Model file for the job. Use its own axes, mm. Face numbers are marked on the shaded views. A direction names the side the tool comes from. Coordinates: 2 decimals unless noted, no trailing zeros. Loops run counter-clockwise (first coordinate to the right, second up) from the corner with the lowest first, then second, coordinate; pieces in that order, holes last.
Autodesk Inventor part; units mm, degrees
ref_plane "YZ Plane" through (0, 0, 0) normal (1, 0, 0) x (0, 1, 0)
ref_plane "XZ Plane" through (0, 0, 0) normal (0, 1, 0) x (-1, 0, 0)
ref_plane "XY Plane" through (0, 0, 0) normal (0, 0, 1) x (1, 0, 0)
sketch "Sketch1" plane through (0, 0, 0) normal (0, 0, 1) x (1, 0, 0)
  line L0 (0, 0) -> (525.78, 0)
  line L1 (0, 0) -> (0, 101.6)
  line L2 (0, 101.6) -> (262.89, 253.3796)
  line L3 (262.89, 253.3796) -> (525.78, 101.6)
  line L4 (525.78, 101.6) -> (525.78, 0)
  line L5 (262.89, 246.0473) -> (6.35, 97.9338)
  line L6 (6.35, 97.9338) -> (6.35, 6.35)
  line L7 (6.35, 6.35) -> (519.43, 6.35)
  line L8 (519.43, 6.35) -> (519.43, 97.9338)
  line L9 (519.43, 97.9338) -> (262.89, 246.0473)
  point P0 (262.89, 0)
  dimension "d0" = 525.78
  dimension "d1" = 101.6
  dimension "d2" = 120
  dimension "d3" = 6.35
extrude "Extrusion1" add sketch "Sketch1" along normal blind 355.6
sketch "Sketch2" plane through (0, 0, 355.6) normal (0, 0, 1) x (1, 0, 0)
  line L0 (262.89, 246.0473) -> (519.43, 97.9338)
  line L1 (519.43, 97.9338) -> (519.43, 6.35)
  line L2 (519.43, 6.35) -> (6.35, 6.35)
  line L3 (6.35, 6.35) -> (6.35, 97.9338)
  line L4 (6.35, 97.9338) -> (262.89, 246.0473)
  line L5 (0, 0) -> (525.78, 0)
  line L6 (525.78, 0) -> (525.78, 101.6)
  line L7 (525.78, 101.6) -> (262.89, 253.3796)
  line L8 (262.89, 253.3796) -> (0, 101.6)
  line L9 (0, 101.6) -> (0, 0)
  circle A0 centre (262.89, 121.3796) radius 60
  dimension "d6" = 120
  dimension "d7" = 132
extrude "Extrusion2" add sketch "Sketch2" along normal blind 6.35 contours L0 L1 L2 L3 L4 | L9 L8 L7 L6 L5
sketch "Sketch3" plane through (0, 0, 0) normal (0, -1, 0) x (1, 0, 0)
  line L0 (0, 0) -> (525.78, 0) construction
  line L1 (525.78, 0) -> (525.78, 88.9)
  line L2 (525.78, 88.9) -> (0, 88.9) construction
  line L3 (0, 88.9) -> (0, 0) construction
  line L4 (86.36, 21.95) -> (86.36, 66.95) construction
  circle A0 centre (86.36, 44.45) radius 2.3812
  circle A1 centre (86.36, 21.95) radius 2.3812
  circle A2 centre (86.36, 66.95) radius 2.3812
  line L5 (146.36, 49.45) -> (146.36, 29.45) construction
  line L6 (156.36, 66.95) -> (156.36, 21.95) construction
  line L7 (146.36, 29.45) -> (166.36, 29.45) construction
  line L8 (166.36, 49.45) -> (146.36, 49.45) construction
  line L9 (86.36, 66.95) -> (226.36, 66.95) construction
  line L10 (226.36, 21.95) -> (86.36, 21.95) construction
  line L11 (86.36, 44.45) -> (226.36, 44.45) construction
  line L12 (166.36, 29.45) -> (166.36, 49.45) construction
  line L13 (226.36, 66.95) -> (226.36, 21.95) construction
  circle A3 centre (226.36, 66.95) radius 2.3813
  circle A4 centre (226.36, 44.45) radius 2.3813
  circle A5 centre (226.36, 21.95) radius 2.3813
  circle A6 centre (156.36, 39.45) radius 10
  line L14 (0, 0) -> (0, 361.95)
  line L15 (525.78, 0) -> (525.78, 361.95)
  line L16 (0, 0) -> (525.78, 0)
  point P0 (0, 44.45)
  point P1 (146.36, 39.45)
  point P2 (166.36, 39.45)
  point P3 (262.89, 0)
  dimension "d10" = 45
  dimension "d11" = 140
  dimension "d12" = 4.7625
  dimension "d13" = 4.7625
  dimension "d14" = 4.7625
  dimension "d15" = 4.7625
  dimension "d16" = 4.7625
  dimension "d17" = 4.7625
  dimension "d18" = 60
  dimension "d19" = 7.5
  dimension "d20" = 20
  dimension "d21" = 20
  dimension "d22" = 86.36
  dimension "d23" = 88.9
extrude "Extrusion3" cut sketch "Sketch3" against normal blind 6.35
sketch "Sketch4" plane through (0, 0, 0) normal (0, -1, 0) x (1, 0, 0)
  line L0 (71.36, 0) -> (241.36, 0)
  line L1 (241.36, 0) -> (241.36, 85)
  line L2 (241.36, 85) -> (71.36, 85)
  line L3 (71.36, 85) -> (71.36, 0)
  line L4 (0, 0) -> (525.78, 0) construction
  circle A0 centre (156.36, 39.45) radius 10 construction
  point P0 (156.36, 85)
  dimension "d26" = 170
  dimension "d27" = 85
extrude "Extrusion4" cut sketch "Sketch4" against normal blind 6.35
sketch "Sketch5" plane through (0, 0, 361.95) normal (0, -1, 0) x (1, 0, 0)
  line L0 (519.43, -6.35) -> (6.35, -6.35)
  line L1 (241.36, -361.95) -> (525.78, -361.95)
  line L2 (0, -361.95) -> (0, 0)
  line L3 (525.78, -361.95) -> (0, -361.95)
  line L4 (0, -361.95) -> (0, -243.4167)
  line L5 (0, -243.4167) -> (525.78, -243.4167)
  line L6 (525.78, -243.4167) -> (525.78, -361.95)
  line L7 (525.78, -243.4167) -> (0, -243.4167)
  line L8 (0, -243.4167) -> (0, -124.8833)
  line L9 (0, -124.8833) -> (525.78, -124.8833)
  line L10 (525.78, -124.8833) -> (525.78, -243.4167)
  line L11 (525.78, -124.8833) -> (0, -124.8833)
  line L12 (0, -124.8833) -> (0, 0)
  line L13 (0, 0) -> (525.78, 0)
  line L14 (525.78, 0) -> (525.78, -124.8833)
  dimension "d30" = 355.6
  dimension "d31" = 118.5333
  dimension "d32" = 118.5333
extrude "Extrusion5" cut sketch "Sketch5" against normal through all contours L5 L2 L9 L10 | L9 L2 L13 L14
equation "\"d31\" = 0.333333 * d30"
equation "\"d32\" = 0.333333 * d30"
properties part number "CA01" material "ABS Plastic"
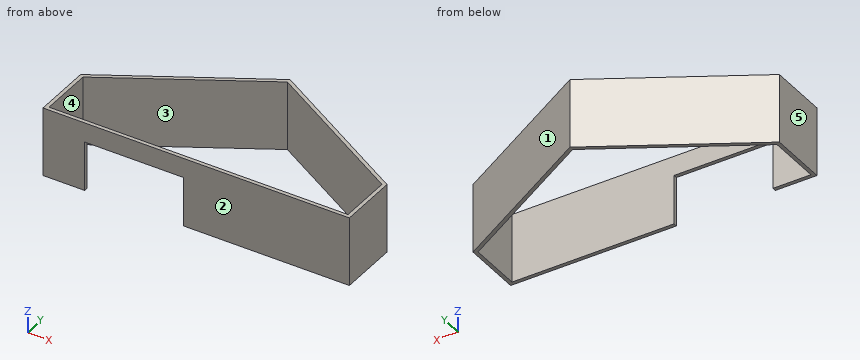
Q1. Slice it at A-A (y = 44). List the corners of the cut face in (x, z), and give its area (3 significant figures).
Answers:
outline: (0, 0) - (6.35, 0) - (6.35, 118.53) - (0, 118.53) - close; (519.43, 0) - (525.78, 0) - (525.78, 118.53) - (519.43, 118.53) - close
area: 1,510 mm2
Q2. Drill centre lines: line 1 (X direction, y = 87.5, z = 26); line 2 (Y direction, x = 408.5, z = 82); line 3 (X direction, y = 128.5, z = 92). Where is each one in solid material? Low to high.
Answers:
line 1: x = 0 to 6.35, 519.43 to 525.78
line 2: y = 0 to 6.35, 161.98 to 169.31
line 3: x = 46.59 to 59.29, 466.49 to 479.19
Q3. Flat gauge pins, fed straight in: P1, Ø5, axis at x = 357, z = 45.5, coming from the +Y side; P2, Ø3, axis at x = 211.5, z = 58, coming from the -Y side; P3, Ø10, axis at x = 202.5, z = 76.5, coming from the +Y side. Where does each tip first touch, or does it go through?
Answers:
P1: stops at y = 200.49
P2: stops at y = 215.51
P3: stops at y = 221.4
Q4. Slice it at D-D (z = 15.5). List the corners of the cut face in (x, y), and give its area (3 significant figures).
Answers:
outline: (0, 0) - (71.36, 0) - (71.36, 6.35) - (6.35, 6.35) - (6.35, 97.93) - (262.89, 246.05) - (519.43, 97.93) - (519.43, 6.35) - (241.36, 6.35) - (241.36, 0) - (525.78, 0) - (525.78, 101.6) - (262.89, 253.38) - (0, 101.6) - close
area: 7,250 mm2
Q5. Which spindle directions (+Z, -Z, +X, -X, +Y, -Y) get a long thin tool onto all of the face, cutting with end or side? Do the marked faces 4 and 5. Say none if no direction does.
Answers:
face 4: +Z, -Z
face 5: +Z, -Z, -X, +Y, -Y
Q6. Slice it at C-C (z = 93.5). List the corners of the cut face in (x, y).
Answers:
outline: (0, 0) - (525.78, 0) - (525.78, 101.6) - (262.89, 253.38) - (0, 101.6) - close; hole (6.35, 6.35) - (519.43, 6.35) - (519.43, 97.93) - (262.89, 246.05) - (6.35, 97.93) - close
Q7. Mould opens along X. For the marked faces 1, 2 and 3 say: +X half, -X half, draft (parallel to the pull), parting line (faces both ways), or undercut.
Answers:
face 1: +X half
face 2: draft
face 3: undercut
Q8. Slice it at B-B (x = 194.5). List the corners of the cut face in (y, z), and give its area (3 significant figures).
Answers:
outline: (0, 85) - (6.35, 85) - (6.35, 118.53) - (0, 118.53) - close; (206.56, 0) - (213.89, 0) - (213.89, 118.53) - (206.56, 118.53) - close
area: 1,080 mm2
